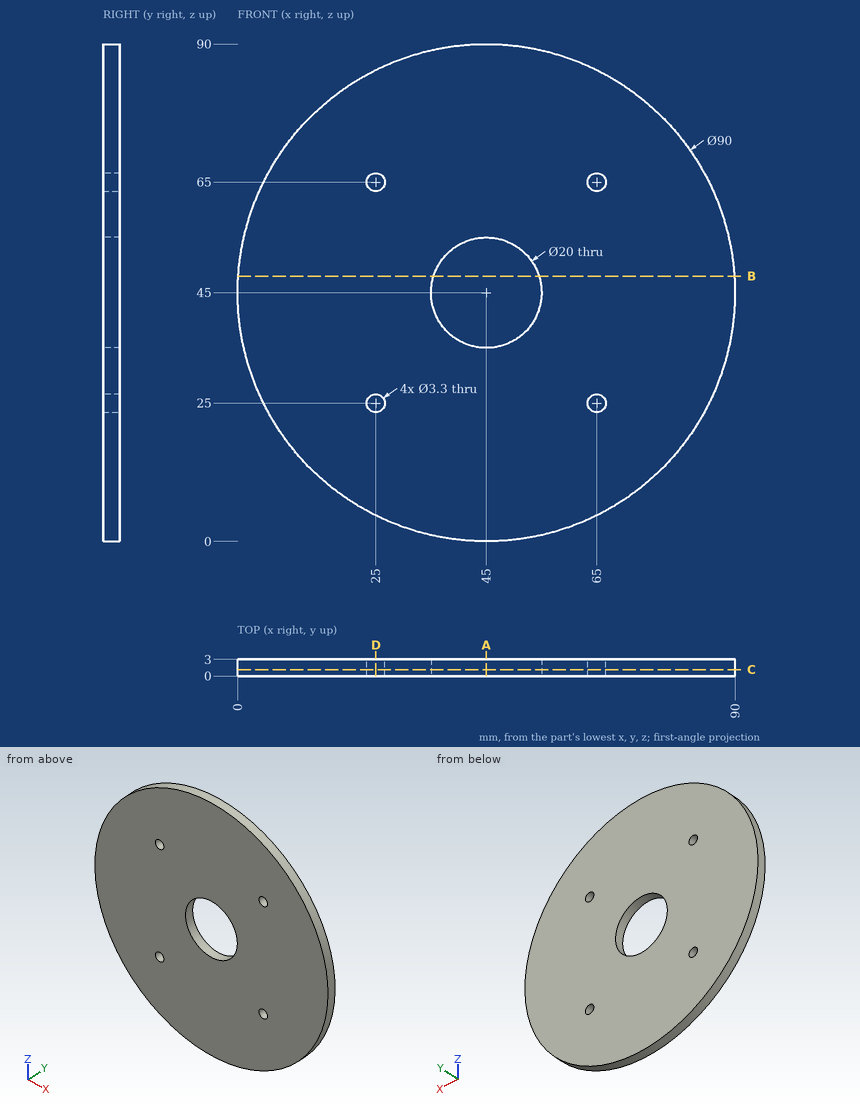
Could you check a few things on this drawing? It's one solid part, dimensions in mm from its lowest x, y, z. Round coordinates to 2 decimals unless told otherwise and drop trailing zeros. Order: outer loops, then holes, each group sorted by start corner. A loop starts at its lowest first (then second) coordinate and runs counter-clockwise, first axis right, second up. Notation, with made-up numbers: M -3.75,-22.75 L 1.25,-22.75 A31 cw 1.25,11.25 Z; hole C 32.5,7 d1. An arc over 180 degrees is marked long. One line per item, written item: value.
(1) Imagine slicing it at B-B (z = 48). Write out the boundary of the cut face in (x, y).
Ans:
outline: M 0.1,0 L 35.46,0 L 35.46,3 L 0.1,3 Z; M 54.54,0 L 89.9,0 L 89.9,3 L 54.54,3 Z
(2) Imagine slicing it at D-D (x = 25). Write out the boundary of the cut face in (y, z), and give its area (3 significant figures).
Ans:
outline: M 0,4.69 L 3,4.69 L 3,23.35 L 0,23.35 Z; M 0,26.65 L 3,26.65 L 3,63.35 L 0,63.35 Z; M 0,66.65 L 3,66.65 L 3,85.31 L 0,85.31 Z
area: 222 mm^2
(3) I'm going to push flat-ended pins straight in: P1, Ø1, axis at y = 2, z = 28, coming from the -X side; P2, Ø2, axis at x = 22, z = 39.5, coming from the -Y side; P3, Ø2.5, axis at x = 25, z = 25, coming from the +Y side; P4, Ø1.5, axis at y = 2.5, z = 15.5, coming from the +X side. Where does each tip first touch, or does it pass through?
Ans:
P1: stops at x = 3.13
P2: stops at y = 0
P3: passes through
P4: stops at x = 79.62
(4) I need wall thicknesses on line 1 along X through (y, z) = (1.95, 66.5); line 2 along X through (y, z) = (1.6, 25.5); line 3 along Z through (x, y) = (65, 1.25). Which ranges of each line are inside material? Lowest first, please. Write a range as from..to.
Ans:
line 1: x = 5.47..24.31, 25.69..64.31, 65.69..84.53
line 2: x = 4.44..23.43, 26.57..63.43, 66.57..85.56
line 3: z = 4.69..23.35, 26.65..63.35, 66.65..85.31
(5) Imagine slicing it at A-A (x = 45). Write out the boundary of the cut face in (y, z).
Ans:
outline: M 0,0 L 3,0 L 3,35 L 0,35 Z; M 0,55 L 3,55 L 3,90 L 0,90 Z
(6) Imagine slicing it at C-C (y = 1.15). Write out the boundary of the cut face in (x, z), and give its area (3 significant figures).
Ans:
outline: C 45,45 d90; hole C 25,25 d3.3; hole C 25,65 d3.3; hole C 45,45 d20; hole C 65,25 d3.3; hole C 65,65 d3.3
area: 6,010 mm^2
